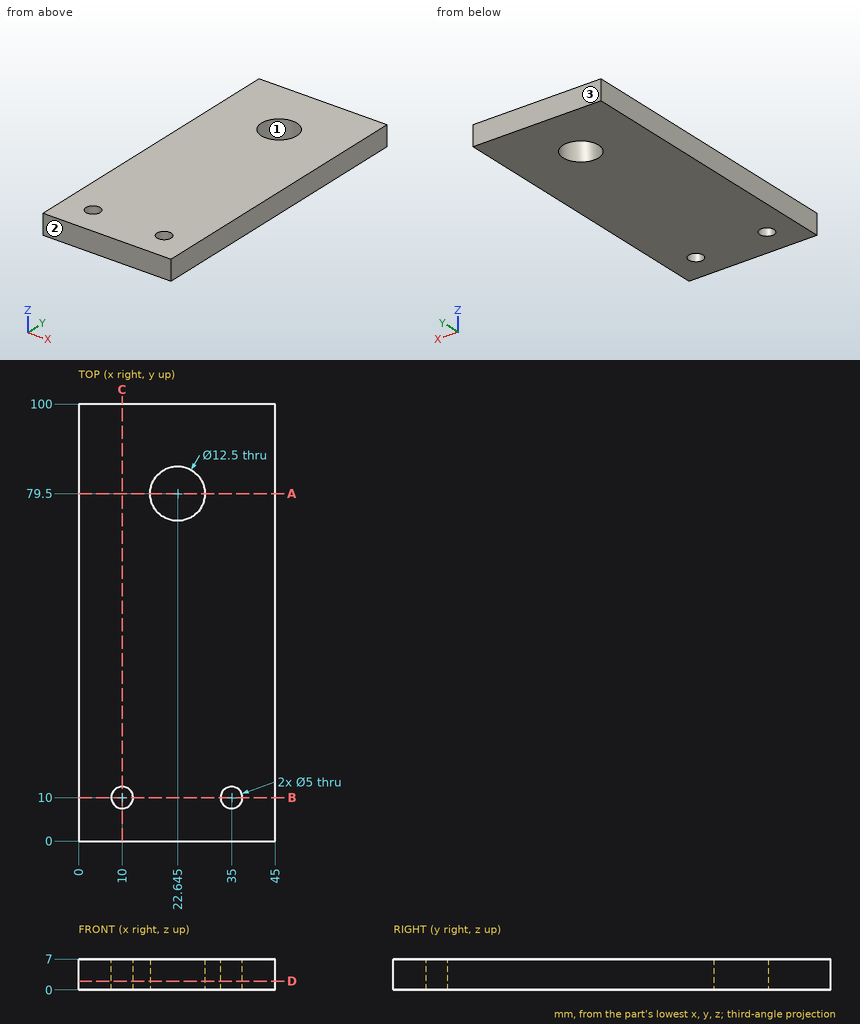
For this review, use the dimensioned drawing (mm, ordinates from the lowest corner) and the shaded views. Coordinates: 2 decimals unless noted, no trailing zeros. Loops run counter-clockwise (first coordinate to the right, second up) from the corner with the lowest first, then second, coordinate; pieces in that order, holes last. Notation, with made-up numbers: (0, -34) -> (51, -34) arc R17 ccw to (51, -27) -> close; hole circle Ø11 at (-21.75, 31). An arc over 180 degrees is marked (long way). Use a Markdown table: item, result. Add a question column.
1. Add section B-B on y = 10. Write out the cut boundary in (x, z).
2. To check wall thickness, follow line 1 (X direction, y = 10, z = 3.75); line 2 (Y direction, x = 10, z = 3.25); line 3 (X direction, y = 79.5, z = 4.5) (1 decimal). State the ranges of each line that lie inside material, in increasing order.
3. Add section D-D on z = 2. Give the number of separate pieces and of enclosed holes in the cut face, plus the area to 3 significant figures.
4. Add section A-A on y = 79.5. Write out the cut boundary in (x, z) (1 decimal).
5. Add section C-C on x = 10. Write out the cut boundary in (y, z).
6. Clearance check with a flat-ended pin moving along its axis: pin 1 Ø4 at (x, z) = (6.5, 4.5) entering from -Y. State where the tip first meets the part, or that it passes through.
7. Draft analysis for pull direction Y (two halves, no side actions). For the marked faces 1, 2 and 3, state which applies: pulls with the +Y half, pulls with the -Y half, needs draft (parallel to the pull), parting line crosses it, or undercut.
Returned:
| question | item | result |
|---|---|---|
| 1 | outline | (0, 0) -> (7.5, 0) -> (7.5, 7) -> (0, 7) -> close; (12.5, 0) -> (32.5, 0) -> (32.5, 7) -> (12.5, 7) -> close; (37.5, 0) -> (45, 0) -> (45, 7) -> (37.5, 7) -> close |
| 2 | line 1 | x = 0 to 7.5, 12.5 to 32.5, 37.5 to 45 |
| 2 | line 2 | y = 0 to 7.5, 12.5 to 100 |
| 2 | line 3 | x = 0 to 16.4, 28.9 to 45 |
| 3 | separate pieces | 1 |
| 3 | enclosed holes | 3 |
| 3 | area | 4,340 mm² |
| 4 | outline | (0, 0) -> (16.4, 0) -> (16.4, 7) -> (0, 7) -> close; (28.9, 0) -> (45, 0) -> (45, 7) -> (28.9, 7) -> close |
| 5 | outline | (0, 0) -> (7.5, 0) -> (7.5, 7) -> (0, 7) -> close; (12.5, 0) -> (100, 0) -> (100, 7) -> (12.5, 7) -> close |
| 6 | pin 1 | stops at y = 0 |
| 7 | face 1 | undercut |
| 7 | face 2 | pulls with the -Y half |
| 7 | face 3 | pulls with the +Y half |
